Part model, mm, in its own coordinate system. Face numbers are marked on the shaded views. Coordinates: 2 decimals unless noted, no trailing zeros. Write each loop counter-clockwise with the first axis right and the second up, starting at its lowest first coordinate (ties: lowest second). Pieces come first, ordered by that corner, then holes. Notation, with made-up numbers: (-6.5, 33.25) - (13.5, 33.25) arc R19 ccw to (13.5, 56.25) - close; hole circle Ø10 at (-15.75, -30). An arc over 180 degrees is marked (long way). Use a Markdown table: item, result.
```python
from build123d import *

# Parameters (mm, degrees)
SKETCH1_R           = 9
BOSS_EXTRUDE1_DEPTH = 65
SKETCH2_R           = 8
CUT_EXTRUDE1_DEPTH  = 0.1


with BuildPart() as part:
    # Sketch1 → Boss-Extrude1 (new body)
    with BuildSketch(Plane(origin=(0, 0, 0), x_dir=(1, 0, 0), z_dir=(0, 1, 0))):
        with Locations(Location((0, 0, 0), (0, 0, 270))):
            Circle(SKETCH1_R)
    extrude(amount=BOSS_EXTRUDE1_DEPTH)

    # Sketch2 → Cut-Extrude1 (cut)
    with BuildSketch(Plane(origin=(0, 65, 0), x_dir=(1, 0, 0), z_dir=(0, 1, 0))):
        with Locations(Location((0, 0, 0), (0, 0, 270))):
            Circle(SKETCH2_R)
    cut_extrude1 = extrude(amount=-CUT_EXTRUDE1_DEPTH, mode=Mode.SUBTRACT)

    # Mirror1: Cut-Extrude1 across plane
    add(cut_extrude1.mirror(Plane.ZX.offset(32.5)), mode=Mode.SUBTRACT)


solid = part.part
```
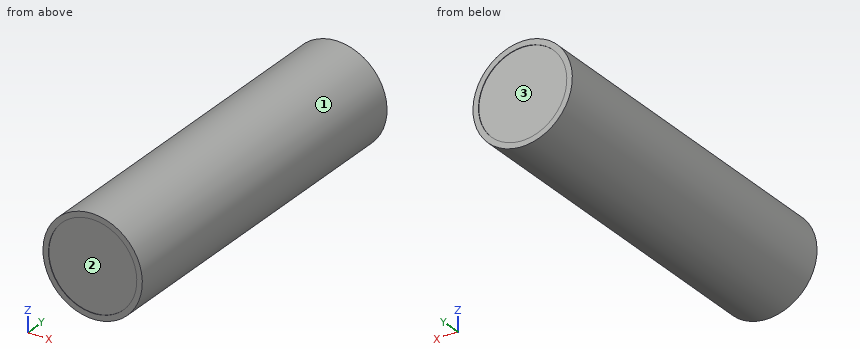
Item 1: Band-saw the part on B-B, the plane z = -3.5. Give the cut face in (x, y).
From the geometry:
| item | result |
|---|---|
| outline | (-8.29, 0) - (-7.19, 0) - (-7.19, 0.1) - (7.19, 0.1) - (7.19, 0) - (8.29, 0) - (8.29, 65) - (7.19, 65) - (7.19, 64.9) - (-7.19, 64.9) - (-7.19, 65) - (-8.29, 65) - close |
Item 2: Band-saw the part on C-C, the plane y = 50. Give the cut face in (x, z), then the cut area to 3 significant figures.
From the geometry:
| item | result |
|---|---|
| outline | circle Ø18 at (0, 0) |
| area | 254 mm^2 |
Item 3: Drop flat-ended pins along their axis: P1, Ø2, axis at x = -4, y = 33.5, coming from the +Z side; P2, Ø1, axis at x = -6.5, y = 57.5, coming from the -Z side; P3, Ø8, axis at x = -0.5, z = -1.5, coming from the +Y side. Give the stop position or say it passes through.
From the geometry:
| item | result |
|---|---|
| P1 | z = 8.49 |
| P2 | z = -6.71 |
| P3 | y = 64.9 |
Item 4: Band-saw the part on A-A, the plane x = -3.5. Give the cut face in (y, z).
From the geometry:
| item | result |
|---|---|
| outline | (0, -8.29) - (65, -8.29) - (65, -7.19) - (64.9, -7.19) - (64.9, 7.19) - (65, 7.19) - (65, 8.29) - (0, 8.29) - (0, 7.19) - (0.1, 7.19) - (0.1, -7.19) - (0, -7.19) - close |
Item 5: Drill centre lines: probe 1 along X at (y, z) = (0.05, 0); probe 2 along Y at (x, z) = (-6.5, 4); probe 3 along X at (y, z) = (38.5, 6.5). Where is each one in solid material? Low to high.
From the geometry:
| item | result |
|---|---|
| probe 1 | -9 to -8, 8 to 9 |
| probe 2 | 0.1 to 64.9 |
| probe 3 | -6.22 to 6.22 |
Item 6: Two-plate mould, pull along Z, no slides. Class the marked faces 1, 2 and 3: pulls with the +Z half, pulls with the -Z half, needs draft (parallel to the pull), parting line crosses it, or undercut.
From the geometry:
| item | result |
|---|---|
| face 1 | parting line crosses it |
| face 2 | undercut |
| face 3 | undercut |
